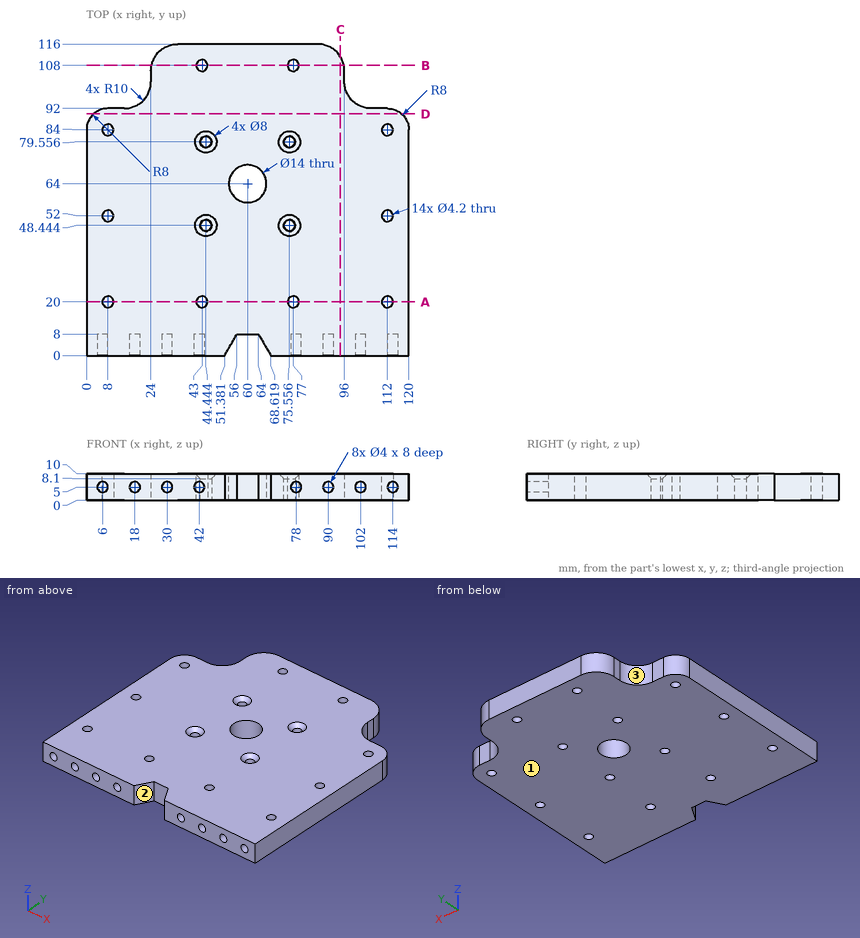
Study the drawing (mm; zero at the part's minimum x, y, z) and answer. Round coordinates to 2 decimals unless told otherwise and drop trailing zeros. Write each loop counter-clockwise with the first axis right and the second up, starting at its lowest first coordinate (ties: lowest second). Pieces come first, ordered by that corner, then holes. Notation, with made-up numbers: (-8.5, -15.75) -> (6.5, -15.75) arc R13 ccw to (6.5, 8.25) -> close; hole circle Ø2 at (-8, -31.75). An arc over 180 degrees is marked (long way). Use CSV: the item, a comma, the result in double quotes. Start each with the question number.
(1) Section D-D on y = 90 is taken. Give the vertices of the cut face in (x, z).
(2) Each of these flat-tipped pins is pushed along its axis until it touches: pin 1 (4 mm diameter, centred on x = 44.44, y = 79.56, fed in from +Z); pin 2 (6 mm diameter, centred on y = 101, z = 1.5, fed in from -X) (1 decimal); pin 3 (1.2 mm diameter, centred on x = 29.5, z = 5.5, fed in from -Y); pin 4 (4.5 mm diameter, centred on y = 105, z = 7, fed in from +X). Where does it stop, or does it pass through?
(3) Section C-C on x = 94.5 is taken. Give the vertices of the cut face in (y, z), then the cut area to 3 significant figures.
(4) Section A-A on y = 20 is taken. Give the vertices of the cut face in (x, z), then the cut area to 3 significant figures.
(5) The mould has two halves that part along X. Classify the marked faces 1, 2 and 3: released by +X, released by -X, zero draft, split by the parting line, or undercut.
(6) Consider L1, parallel to Y at x = 112, z = 3; L2, parallel to Y at x = 78.5, z = 8.25; L3, parallel to X at y = 85, z = 5.5. Determine where each line is inside the solid, lowest interval first. Write a range as from..to.
(7) Section B-B on y = 108 is taken. Give the vertices of the cut face in (x, z).
A:
1,outline,"(2.71, 0) -> (117.29, 0) -> (117.29, 10) -> (2.71, 10) -> close"
2,pin 1,"passes through"
2,pin 2,"stops at x = 23.2"
2,pin 3,"stops at y = 8"
2,pin 4,"stops at x = 96"
3,outline,"(0, 0) -> (111.27, 0) -> (111.27, 10) -> (0, 10) -> close"
3,area,"1,110 mm²"
4,outline,"(0, 0) -> (5.9, 0) -> (5.9, 10) -> (0, 10) -> close; (10.1, 0) -> (40.9, 0) -> (40.9, 10) -> (10.1, 10) -> close; (45.1, 0) -> (74.9, 0) -> (74.9, 10) -> (45.1, 10) -> close; (79.1, 0) -> (109.9, 0) -> (109.9, 10) -> (79.1, 10) -> close; (114.1, 0) -> (120, 0) -> (120, 10) -> (114.1, 10) -> close"
4,area,"1,030 mm²"
5,face 1,"zero draft"
5,face 2,"undercut"
5,face 3,"released by -X"
6,L1,"y = 0..17.9, 22.1..49.9, 54.1..81.9, 86.1..92"
6,L2,"y = 0..18.53, 21.47..106.53, 109.47..116"
6,L3,"x = 0.06..6.15, 9.85..110.15, 113.85..119.94"
7,outline,"(24.2, 0) -> (40.9, 0) -> (40.9, 10) -> (24.2, 10) -> close; (45.1, 0) -> (74.9, 0) -> (74.9, 10) -> (45.1, 10) -> close; (79.1, 0) -> (95.8, 0) -> (95.8, 10) -> (79.1, 10) -> close"
